The listing builds one solid part. Answer for the finished solid, in the listing's coordinates (mm). A direction names the side the tool comes from. Coordinates: 2 decimals unless noted, no trailing zeros. Order: outer loops, then holes, each group sorted by start corner. A loop starts at its lowest first (then second) coordinate and runs counter-clockwise, first axis right, second up. Notation, with made-up numbers: (-7.5, -20) -> (28.5, -20) arc R15 ccw to (28.5, 5) -> close; hole circle Ø5 at (14, 3.5). An arc over 180 degrees is marked (long way). Return JSON: item names as keys, results as strings.
from build123d import *

# Parameters (mm, degrees)
SKETCH1_W           = 145
SKETCH1_H           = 25
BOSS_EXTRUDE1_DEPTH = 10
SKETCH2_W           = 17.5
SKETCH2_H           = 32
BOSS_EXTRUDE2_DEPTH = 10
SKETCH4_W           = 73.5
SKETCH4_H           = 32
BOSS_EXTRUDE3_DEPTH = 10
SKETCH8_R           = 2.25
CUT_EXTRUDE5_DEPTH  = 193.888568868
SKETCH9_W           = 7.3
SKETCH9_H           = 4
CUT_EXTRUDE6_DEPTH  = 10
CUT_EXTRUDE7_REACH  = 195.92
SKETCH10_R          = 3.65
SKETCH11_R          = 12.75
CUT_EXTRUDE8_DEPTH  = 7
CUT_EXTRUDE9_REACH  = 196.692
SKETCH12_R          = 1.75
CUT_EXTRUDE10_DEPTH = 3
CUT_EXTRUDE11_REACH = 196.098
SKETCH14_R          = 1.65
CHAMFER1_SIZE       = 1.5
CHAMFER1_SIZE2      = 0.866025404
FILLET1_R           = 15


with BuildPart() as part:
    # Sketch1 → Boss-Extrude1 (new body)
    with BuildSketch(Plane(origin=(0, 0, 0), x_dir=(1, 0, 0), z_dir=(0, 1, 0))):
        with Locations((72.5, 12.5)):
            Rectangle(SKETCH1_W, SKETCH1_H)
    extrude(amount=BOSS_EXTRUDE1_DEPTH)

    # Sketch2 → Boss-Extrude2 (add)
    with BuildSketch(Plane(origin=(0, 10, 0), x_dir=(1, 0, 0), z_dir=(0, 1, 0))):
        with Locations((153.75, 16)):
            Rectangle(SKETCH2_W, SKETCH2_H)
    extrude(amount=-BOSS_EXTRUDE2_DEPTH)

    # Sketch4 → Boss-Extrude3 (add)
    with BuildSketch(Plane.XZ):
        with Locations((154.25, -16)):
            Rectangle(SKETCH4_W, SKETCH4_H)
    extrude(amount=BOSS_EXTRUDE3_DEPTH)

    # Sketch8 → Cut-Extrude5 (cut, through all)
    with BuildSketch(Plane(origin=(0, 0, -25), x_dir=(-1, 0, 0), z_dir=(0, 0, -1))):
        with Locations((-137, 5)):
            Circle(SKETCH8_R)
        with Locations((-123, 5)):
            Circle(SKETCH8_R)
        with Locations(Location((-22, 5, 0), (0, 0, 180))):
            Circle(SKETCH8_R)
        with Locations(Location((-8, 5, 0), (0, 0, 180))):
            Circle(SKETCH8_R)
    extrude(amount=-CUT_EXTRUDE5_DEPTH, mode=Mode.SUBTRACT)

    # Sketch9 → Cut-Extrude6 (cut)
    with BuildSketch(Plane(origin=(0, 10, 0), x_dir=(1, 0, 0), z_dir=(0, 1, 0))):
        with Locations((137, 20)):
            Rectangle(SKETCH9_W, SKETCH9_H)
        with Locations((137, 5)):
            Rectangle(SKETCH9_W, SKETCH9_H)
        with Locations((123, 5)):
            Rectangle(SKETCH9_W, SKETCH9_H)
        with Locations((123, 20)):
            Rectangle(SKETCH9_W, SKETCH9_H)
        with Locations((8, 20)):
            Rectangle(SKETCH9_W, SKETCH9_H)
        with Locations((22, 20)):
            Rectangle(SKETCH9_W, SKETCH9_H)
        with Locations((22, 5)):
            Rectangle(SKETCH9_W, SKETCH9_H)
        with Locations((8, 5)):
            Rectangle(SKETCH9_W, SKETCH9_H)
    extrude(amount=-CUT_EXTRUDE6_DEPTH, mode=Mode.SUBTRACT)

    # Sketch10 → Cut-Extrude7 (cut, up to next)
    with BuildSketch(Plane(origin=(0, 0, 0), x_dir=(1, 0, 0), z_dir=(0, 1, 0)), mode=Mode.PRIVATE) as cut_extrude7_sk1:
        with Locations(Location((176, 16, 0), (0, 0, 270))):
            Circle(SKETCH10_R)
    cut_extrude7_tool1 = extrude(cut_extrude7_sk1.sketch, amount=-CUT_EXTRUDE7_REACH, mode=Mode.PRIVATE) & part.part
    add(cut_extrude7_tool1.solids().sort_by_distance((176, 0, -16))[0], mode=Mode.SUBTRACT)

    # Sketch11 → Cut-Extrude8 (cut)
    with BuildSketch(Plane.XZ.offset(10)):
        with Locations(Location((176, -16, 0), (0, 0, 270))):
            Circle(SKETCH11_R)
    extrude(amount=-CUT_EXTRUDE8_DEPTH, mode=Mode.SUBTRACT)

    # Sketch12 → Cut-Extrude9 (cut, up to next)
    with BuildSketch(Plane(origin=(0, 10, 0), x_dir=(1, 0, 0), z_dir=(0, 1, 0)), mode=Mode.PRIVATE) as cut_extrude9_sk1:
        with Locations(Location((47.25, 12.5, 0), (0, 0, 270))):
            Circle(SKETCH12_R)
    cut_extrude9_tool1 = extrude(cut_extrude9_sk1.sketch, amount=-CUT_EXTRUDE9_REACH, mode=Mode.PRIVATE) & part.part
    # Sketch12 → Cut-Extrude9 (cut, up to next)
    with BuildSketch(Plane(origin=(0, 10, 0), x_dir=(1, 0, 0), z_dir=(0, 1, 0)), mode=Mode.PRIVATE) as cut_extrude9_sk2:
        with Locations(Location((72.5, 12.5, 0), (0, 0, 270))):
            Circle(SKETCH12_R)
    cut_extrude9_tool2 = extrude(cut_extrude9_sk2.sketch, amount=-CUT_EXTRUDE9_REACH, mode=Mode.PRIVATE) & part.part
    # Sketch12 → Cut-Extrude9 (cut, up to next)
    with BuildSketch(Plane(origin=(0, 10, 0), x_dir=(1, 0, 0), z_dir=(0, 1, 0)), mode=Mode.PRIVATE) as cut_extrude9_sk3:
        with Locations(Location((97.75, 12.5, 0), (0, 0, 270))):
            Circle(SKETCH12_R)
    cut_extrude9_tool3 = extrude(cut_extrude9_sk3.sketch, amount=-CUT_EXTRUDE9_REACH, mode=Mode.PRIVATE) & part.part
    add(cut_extrude9_tool1.solids().sort_by_distance((47.25, 10, -12.5))[0], mode=Mode.SUBTRACT)
    add(cut_extrude9_tool2.solids().sort_by_distance((72.5, 10, -12.5))[0], mode=Mode.SUBTRACT)
    add(cut_extrude9_tool3.solids().sort_by_distance((97.75, 10, -12.5))[0], mode=Mode.SUBTRACT)

    # Sketch13 → Cut-Extrude10 (cut)
    with BuildSketch(Plane(origin=(0, 10, 0), x_dir=(1, 0, 0), z_dir=(0, 1, 0))):
        Polygon((75.964101615, 12.5), (74.232050808, 15.5), (70.767949192, 15.5), (69.035898385, 12.5), (70.767949192, 9.5), (74.232050808, 9.5), align=None)
        Polygon((50.714101615, 12.5), (48.982050808, 15.5), (45.517949192, 15.5), (43.785898385, 12.5), (45.517949192, 9.5), (48.982050808, 9.5), align=None)
        Polygon((101.214101615, 12.5), (99.482050808, 15.5), (96.017949192, 15.5), (94.285898385, 12.5), (96.017949192, 9.5), (99.482050808, 9.5), align=None)
    extrude(amount=-CUT_EXTRUDE10_DEPTH, mode=Mode.SUBTRACT)

    # Sketch14 → Cut-Extrude11 (cut, up to next)
    with BuildSketch(Plane.XZ.offset(3), mode=Mode.PRIVATE) as cut_extrude11_sk1:
        with Locations(Location((176, -7.5, 0), (0, 0, 270))):
            Circle(SKETCH14_R)
    cut_extrude11_tool1 = extrude(cut_extrude11_sk1.sketch, amount=-CUT_EXTRUDE11_REACH, mode=Mode.PRIVATE) & part.part
    # Sketch14 → Cut-Extrude11 (cut, up to next)
    with BuildSketch(Plane.XZ.offset(3), mode=Mode.PRIVATE) as cut_extrude11_sk2:
        with Locations(Location((176, -24.5, 0), (0, 0, 270))):
            Circle(SKETCH14_R)
    cut_extrude11_tool2 = extrude(cut_extrude11_sk2.sketch, amount=-CUT_EXTRUDE11_REACH, mode=Mode.PRIVATE) & part.part
    add(cut_extrude11_tool1.solids().sort_by_distance((176, -3, -7.5))[0], mode=Mode.SUBTRACT)
    add(cut_extrude11_tool2.solids().sort_by_distance((176, -3, -24.5))[0], mode=Mode.SUBTRACT)

    # Chamfer1
    chamfer1_edges = [part.edges().sort_by_distance(p)[0] for p in [
        (176, 0, -5.85),
        (176, 0, -22.85),
    ]]
    chamfer1_side = [part.faces().sort_by_distance(p)[0] for p in [
        (162.928514877, 0, -16),
    ]]
    chamfer(chamfer1_edges, length=CHAMFER1_SIZE, length2=CHAMFER1_SIZE2, reference=chamfer1_side[0])

    # Fillet1
    fillet1_edges = [part.edges().sort_by_distance(p)[0] for p in [
        (162.5, 5, -32),
        (162.5, 5, 0),
        (191, -5, -32),
        (191, -5, 0),
    ]]
    fillet(fillet1_edges, radius=FILLET1_R)


solid = part.part
1. The part is cut by section A-A on x = 22. Give the vertices of the cut face in (y, z), and give its area (3 significant figures).
Answer block:
{"outline": "(0, -25) -> (2.75, -25) -> (2.75, -22) -> (0, -22) -> close; (0, -18) -> (2.75, -18) -> (2.75, -7) -> (0, -7) -> close; (0, -3) -> (2.75, -3) -> (2.75, 0) -> (0, 0) -> close; (7.25, -25) -> (10, -25) -> (10, -22) -> (7.25, -22) -> close; (7.25, -18) -> (10, -18) -> (10, -7) -> (7.25, -7) -> close; (7.25, -3) -> (10, -3) -> (10, 0) -> (7.25, 0) -> close", "area": "93.5 mm2"}
2. The part is cut by section D-D on x = 170. Give the vertices of the cut face in (y, z), and give its area (4 significant figures).
Answer block:
{"outline": "(-10, -32) -> (0, -32) -> (0, 0) -> (-10, 0) -> (-10, -4.75) -> (-3, -4.75) -> (-3, -27.25) -> (-10, -27.25) -> close", "area": "162.5 mm2"}
3. Each of these flat-tipped pins is pushed along its axis until it touches: pin 1 Ø6 at (y, z) = (-4.5, -20.5) entering from +X; pin 2 Ø2 at (x, z) = (138, -20) entering from +Y; pin 3 Ø4 at (x, z) = (97.75, -12.5) entering from +Y; pin 4 Ø2.5 at (x, y) = (123, 5) entering from -Z. Where does it stop, or does it pass through?
Answer block:
{"pin 1": "stops at x = 190.99", "pin 2": "stops at y = 0", "pin 3": "stops at y = 7", "pin 4": "passes through"}
4. The part is cut by section C-C on x = 47.25. Give the vertices of the cut face in (y, z).
Answer block:
{"outline": "(0, -25) -> (10, -25) -> (10, -15.5) -> (7, -15.5) -> (7, -14.25) -> (0, -14.25) -> close; (0, -10.75) -> (7, -10.75) -> (7, -9.5) -> (10, -9.5) -> (10, 0) -> (0, 0) -> close"}
5. The part is cut by section B-B on x = 123. Give the vertices of the cut face in (y, z), and give its area (4 significant figures).
Answer block:
{"outline": "(-10, -32) -> (0, -32) -> (0, -25) -> (2.75, -25) -> (2.75, -22) -> (0, -22) -> (0, -18) -> (2.75, -18) -> (2.75, -7) -> (0, -7) -> (0, -3) -> (2.75, -3) -> (2.75, 0) -> (-10, 0) -> close; (7.25, -25) -> (10, -25) -> (10, -22) -> (7.25, -22) -> close; (7.25, -18) -> (10, -18) -> (10, -7) -> (7.25, -7) -> close; (7.25, -3) -> (10, -3) -> (10, 0) -> (7.25, 0) -> close", "area": "413.5 mm2"}
6. Consider line 1 (Z direction, x = 120.5, y = 4); line 2 (Y direction, x = 123, z = -10); line 3 (Y direction, x = 8, z = -24.25). Determine where each line is inside the solid, lowest interval first. Write a range as from..to.
Answer block:
{"line 1": "z = -25..-22, -18..-7, -3..0", "line 2": "y = -10..2.75, 7.25..10", "line 3": "y = 0..2.75, 7.25..10"}
7. Determine the mould class of faces 1 (the face through (24.146, 4.324, -1.521)), 2 (the face through (44.64, 8.52, -11.02)), 3 (the face through (158.22, 4.93, -27.49)) for opening direction Z: pulls with the +Z half, pulls with the -Z half, needs draft (parallel to the pull), parting line crosses it, or undercut.
Answer block:
{"face 1": "needs draft", "face 2": "undercut", "face 3": "pulls with the -Z half"}
8. For faces 4 (the face through (137.8, 7.3, -7)), 5 (the face through (11.65, 5, -20)), 6 (the face through (188.64, -6.55, -14.34)), determine the directions among +Z, -Z, +X, -X, +Y, -Y from which every point of the face is accessible in a straight line to the end or side of a thin tool.
Answer block:
{"face 4": "+Y", "face 5": "+Y, -Y", "face 6": "-Y"}
